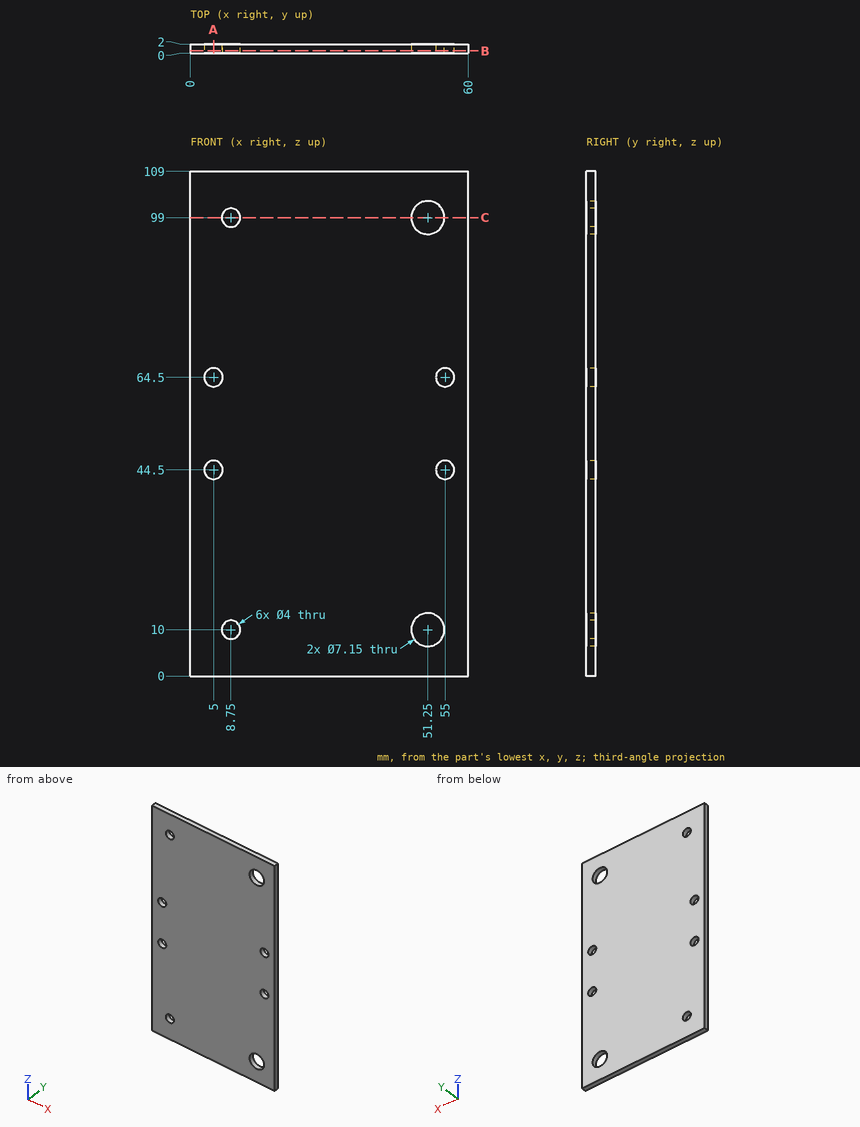
Study the drawing (mm; zero at the part's minimum x, y, z) and answer. Round coordinates to 2 decimals unless told otherwise and drop trailing zeros. Write each loop counter-clockwise with the first axis right and the second up, starting at its lowest first coordinate (ties: lowest second). Pieces come first, ordered by that corner, then holes.
Q1. Straight lines are drawn through the part: line 1 (X direction, y = 0.7, z = 64.5); line 2 (Z direction, x = 5, y = 0.45); line 3 (Z direction, x = 51.25, y = 0.95) (3 decimals). For each, find the intervals that lie inside material, in ascending order.
Values:
line 1: x = 0 to 3, 7 to 53, 57 to 60
line 2: z = 0 to 42.5, 46.5 to 62.5, 66.5 to 109
line 3: z = 0 to 6.425, 13.575 to 95.425, 102.575 to 109
Q2. A flat-ended cylindrical pin translates along its axis: P1, Ø4.5, axis at x = 55, z = 64.5, coming from the -Y side. Find the tip coordinate at first contact, or state that the pin passes through.
Values:
P1: stops at y = 0
Q3. Find section A-A on x = 5. Determine the outline of the cut face in (y, z).
Values:
outline: (0, 0) - (2, 0) - (2, 42.5) - (0, 42.5) - close; (0, 46.5) - (2, 46.5) - (2, 62.5) - (0, 62.5) - close; (0, 66.5) - (2, 66.5) - (2, 109) - (0, 109) - close
Q4. Find section C-C on z = 99. Determine the outline of the cut face in (x, y) (3 decimals), and give its area (3 significant figures).
Values:
outline: (0, 0) - (6.75, 0) - (6.75, 2) - (0, 2) - close; (10.75, 0) - (47.675, 0) - (47.675, 2) - (10.75, 2) - close; (54.825, 0) - (60, 0) - (60, 2) - (54.825, 2) - close
area: 97.7 mm2
Q5. Find section B-B on y = 0.5. State how many separate pieces and enclosed holes the cut face has, and give its area (3 significant figures).
Values:
separate pieces: 1
enclosed holes: 8
area: 6,380 mm2
